from build123d import *

# Parameters (mm, degrees)
SKETCH1_R           = 45
BOSS_EXTRUDE2_DEPTH = 1.5
SKETCH1_5_R         = 45
SKETCH1_5_R_2       = 15
SKETCH1_5_R_3       = 8
BOSS_EXTRUDE3_DEPTH = 1
SKETCH1_6_R         = 15
BOSS_EXTRUDE4_DEPTH = 1.5


with BuildPart() as part:
    # Sketch1 → Boss-Extrude2 (new body, symmetric)
    with BuildSketch(Plane.XY):
        Polygon((-16.176190319, 60.370364143), (-15.625, 58.313293868), (0, 62.5), (0, 60.370364143), (16.176190319, 60.370364143), (15.625, 58.313293868), (31.25, 54.126587737), (30.185182072, 52.282268984), (44.194173824, 44.194173824), (42.688293868, 42.688293868), (54.126587737, 31.25), (52.282268984, 30.185182072), (60.370364143, 16.176190319), (58.313293868, 15.625), (62.5, 0), (60.370364143, 0), (60.370364143, -16.176190319), (58.313293868, -15.625), (54.126587737, -31.25), (52.282268984, -30.185182072), (44.194173824, -44.194173824), (42.688293868, -42.688293868), (31.25, -54.126587737), (30.185182072, -52.282268984), (16.176190319, -60.370364143), (15.625, -58.313293868), (0, -62.5), (0, -60.370364143), (-16.176190319, -60.370364143), (-15.625, -58.313293868), (-31.25, -54.126587737), (-30.185182072, -52.282268984), (-44.194173824, -44.194173824), (-42.688293868, -42.688293868), (-54.126587737, -31.25), (-52.282268984, -30.185182072), (-60.370364143, -16.176190319), (-58.313293868, -15.625), (-62.5, 0), (-60.370364143, 0), (-60.370364143, 16.176190319), (-58.313293868, 15.625), (-54.126587737, 31.25), (-52.282268984, 30.185182072), (-44.194173824, 44.194173824), (-42.688293868, 42.688293868), (-31.25, 54.126587737), (-30.185182072, 52.282268984), align=None)
        Circle(SKETCH1_R, mode=Mode.SUBTRACT)
    extrude(amount=BOSS_EXTRUDE2_DEPTH, both=True)

    # Sketch1_5 → Boss-Extrude3 (add, symmetric)
    with BuildSketch(Plane.XY):
        Circle(SKETCH1_5_R)
        Circle(SKETCH1_5_R_2, mode=Mode.SUBTRACT)
        with Locations((-25.980762114, 15)):
            Circle(SKETCH1_5_R_3, mode=Mode.SUBTRACT)
        with Locations((-25.980762114, -15)):
            Circle(SKETCH1_5_R_3, mode=Mode.SUBTRACT)
        with Locations((0, -30)):
            Circle(SKETCH1_5_R_3, mode=Mode.SUBTRACT)
        with Locations((25.980762114, -15)):
            Circle(SKETCH1_5_R_3, mode=Mode.SUBTRACT)
        with Locations((25.980762114, 15)):
            Circle(SKETCH1_5_R_3, mode=Mode.SUBTRACT)
        with Locations((0, 30)):
            Circle(SKETCH1_5_R_3, mode=Mode.SUBTRACT)
    extrude(amount=BOSS_EXTRUDE3_DEPTH, both=True)

    # Sketch1_6 → Boss-Extrude4 (add, symmetric)
    with BuildSketch(Plane.XY):
        Circle(SKETCH1_6_R)
        with BuildLine():
            ThreePointArc((-3, 8.485281374), (0, -9), (3, 8.485281374))
            Line((3, 8.485281374), (3, 10.485281374))
            Line((3, 10.485281374), (-3, 10.485281374))
            Line((-3, 10.485281374), (-3, 8.485281374))
        make_face(mode=Mode.SUBTRACT)
    extrude(amount=BOSS_EXTRUDE4_DEPTH, both=True)


solid = part.part
CAD build for the part. Positions are in the model's coordinates, mm. A direction names the side the tool comes from. Coordinates: 2 decimals unless noted, no trailing zeros. Order: outer loops, then holes, each group sorted by start corner. A loop starts at its lowest first (then second) coordinate and runs counter-clockwise, first axis right, second up. Notation, with made-up numbers: (16, -20.75) -> (64, -20.75) arc R29 ccw to (64, 14.25) -> close; hole circle Ø1 at (13.5, -26.5). An arc over 180 degrees is marked (long way). Answer in a Markdown table with one row per item.
1) Band-saw the part on C-C (y = 41). List the corners of the cut face in (x, z).
Check values:
| item | result |
|---|---|
| outline | (-46.04, -1.5) -> (-18.55, -1.5) -> (-18.55, -1) -> (18.55, -1) -> (18.55, -1.5) -> (44.38, -1.5) -> (44.38, 1.5) -> (18.55, 1.5) -> (18.55, 1) -> (-18.55, 1) -> (-18.55, 1.5) -> (-46.04, 1.5) -> close |
2) Flat gauge pins, fed straight in: P1, Ø10, axis at x = -27.5, y = 19, coming from the +Z side; P2, Ø1.7, axis at y = -62, z = 0.5, coming from the -X side; P3, Ø1.5, axis at y = 2, z = -1, coming from the +X side. Where does each tip first touch, or does it go through?
Check values:
| item | result |
|---|---|
| P1 | z = 1 |
| P2 | x = 0 |
| P3 | x = 62.17 |
3) Drill centre lines: line 1 (X direction, y = 11, z = 0.65); line 2 (Y direction, x = 6, z = -0.1); line 3 (Y direction, x = -24.5, z = -0.05). Where is each one in solid material? Low to high.
Check values:
| item | result |
|---|---|
| line 1 | -60.37 to -32.91, -19.05 to 19.05, 32.91 to 59.55 |
| line 2 | -60.89 to -35.29, -24.71 to -6.71, 6.71 to 24.71, 35.29 to 60.37 |
| line 3 | -55.94 to -22.86, -7.14 to 7.14, 22.86 to 55.56 |
4) Band-saw the part on B-B (y = -12). List the corners of the cut face in (x, z), and give its area (3 significant figures).
Check values:
| item | result |
|---|---|
| outline | (-59.28, -1.5) -> (-43.37, -1.5) -> (-43.37, -1) -> (-33.4, -1) -> (-33.4, 1) -> (-43.37, 1) -> (-43.37, 1.5) -> (-59.28, 1.5) -> close; (-18.56, -1) -> (-9, -1) -> (-9, -1.5) -> (9, -1.5) -> (9, -1) -> (18.56, -1) -> (18.56, 1) -> (9, 1) -> (9, 1.5) -> (-9, 1.5) -> (-9, 1) -> (-18.56, 1) -> close; (33.4, -1) -> (43.37, -1) -> (43.37, -1.5) -> (60.37, -1.5) -> (60.37, 1.5) -> (43.37, 1.5) -> (43.37, 1) -> (33.4, 1) -> close |
| area | 231 mm2 |
5) Band-saw the part on D-D (z = 0.4). Give the number of separate pieces and of enclosed holes in the cut face, and give its area (3 significant figures).
Check values:
| item | result |
|---|---|
| separate pieces | 1 |
| enclosed holes | 7 |
| area | 10,200 mm2 |
6) Mould opens along Y. For faces 4 (the face through (-11, 11, -1)), 5 (the face through (56.25, -23.33, 0.02)), 6 (the face through (-7.922, 60.377, 0.021)) say: pulls with the +Y half, pulls with the -Y half, needs draft (parallel to the pull), parting line crosses it, or undercut.
Check values:
| item | result |
|---|---|
| face 4 | undercut |
| face 5 | pulls with the -Y half |
| face 6 | pulls with the +Y half |
7) Band-saw the part on A-A (x = -23). List the corners of the cut face in (y, z).
Check values:
| item | result |
|---|---|
| outline | (-56.34, -1.5) -> (-38.68, -1.5) -> (-38.68, -1) -> (-22.42, -1) -> (-22.42, 1) -> (-38.68, 1) -> (-38.68, 1.5) -> (-56.34, 1.5) -> close; (-7.58, -1) -> (7.58, -1) -> (7.58, 1) -> (-7.58, 1) -> close; (22.42, -1) -> (38.68, -1) -> (38.68, -1.5) -> (56.43, -1.5) -> (56.43, 1.5) -> (38.68, 1.5) -> (38.68, 1) -> (22.42, 1) -> close |
8) Which spindle directions (+Z, -Z, +X, -X, +Y, -Y) get a long thin tool onto all of the face, cutting with end or side? Do faces 1 (the face through (60.377, 7.922, 0.021)), 2 (the face through (-23.28, 56.27, 0.02)), 3 (the face through (-14.985, 0.66, 1.254)). Say none if no direction does.
Check values:
| item | result |
|---|---|
| face 1 | +Z, -Z, +X |
| face 2 | +Z, -Z, +Y |
| face 3 | +Z |
